Autodesk Inventor part; units mm, degrees
ref_plane "YZ Plane" through (0, 0, 0) normal (1, 0, 0) x (0, 1, 0)
ref_plane "XZ Plane" through (0, 0, 0) normal (0, 1, 0) x (-1, 0, 0)
ref_plane "XY Plane" through (0, 0, 0) normal (0, 0, 1) x (1, 0, 0)
sketch "スケッチ1" plane through (0, 0, 0) normal (1, 0, 0) x (0, 1, 0)
  line L0 (0, -1) -> (0, 6) construction
  line L1 (6, 5) -> (7, 5)
  line L2 (7, 5) -> (7, 0)
  line L3 (7, 0) -> (6, 0)
  line L4 (6, 0) -> (6, 5)
  line L5 (7, 1) -> (9, 1)
  line L6 (9, 1) -> (9, 0)
  line L7 (9, 0) -> (7, 0)
  line L8 (7, 0) -> (7, 1)
  point P0 (0, 0)
  point P1 (7, 0)
  dimension "d0" = 12
  dimension "d1" = 14
  dimension "d10" = 5
  dimension "d14" = 1
  dimension "d15" = 18
revolve "回転1" add sketch "スケッチ1" angle 360 about axis through (0, 0, -10) along (0, 0, 1)
chamfer "面取り1" distance 0.5 angle 30 1 edges at (0, -7, 5) measured on face at (0.5633, 6.9773, 2.3333)
fillet "フィレット2" radius 0.5 1 edges at (0, -7, 1)
properties part number "_GFM-0608-04" material "アセタール樹脂、黒"
Design review of the part built by this model. Coordinates are the model's own, in mm. Coordinates: 2 decimals unless noted, no trailing zeros. Order: outer loops, then holes, each group sorted by start corner. A loop starts at its lowest first (then second) coordinate and runs counter-clockwise, first axis right, second up.
Item 1: Take a section at C-C, the plane z = 0.6. Write out the cut boundary in (x, y), then the cut area to 3 significant figures.
Item 2: Take a section at D-D, the plane z = 3.8. Write out the cut boundary in (x, y).
Item 3: For pin 1 Ø2 at (y, z) = (-4, 1.5) entering from -X, flat-tipped, find the tip position at first contact; note if it passes through.
Item 4: For line 1 (X direction, y = 0, z = 2.75); line 2 (Y direction, x = 0.25, z = 0.8), list the stretches that pass through material, from the lowest coordinate up.
Item 5: Take a section at A-A, the plane y = 0. Write out the cut boundary in (x, z), then the cut area to 3 significant figures.
Item 6: The part is to be moulded in two halves that separate along Y. For faces 1 (the cylindrical face through (0, -6, 3)), 2 (the flat face through (-7.4, -2, 1)), 3 (the cylindrical face through (-2.681, 6.466, 2.979)), say which applies: pulls with the +Y half, pulls with the -Y half, needs draft (parallel to the pull), parting line crosses it, or undercut.
The answers:
1. outline: circle Ø18 at (0, 0); hole circle Ø12 at (0, 0)
1. area: 141 mm2
2. outline: circle Ø14 at (0, 0); hole circle Ø12 at (0, 0)
3. pin 1: stops at x = -8.44
4. line 1: x = -7 to -6, 6 to 7
4. line 2: y = -9 to -5.99, 5.99 to 9
5. outline: (-9, 0) - (-6, 0) - (-6, 5) - (-6.71, 5) - (-7, 4.5) - (-7, 1.5) arc R0.5 cw to (-7.5, 1) - (-9, 1) - close; (6, 0) - (9, 0) - (9, 1) - (7.5, 1) arc R0.5 cw to (7, 1.5) - (7, 4.5) - (6.71, 5) - (6, 5) - close
5. area: 14.0 mm2
6. face 1: undercut
6. face 2: needs draft
6. face 3: parting line crosses it
